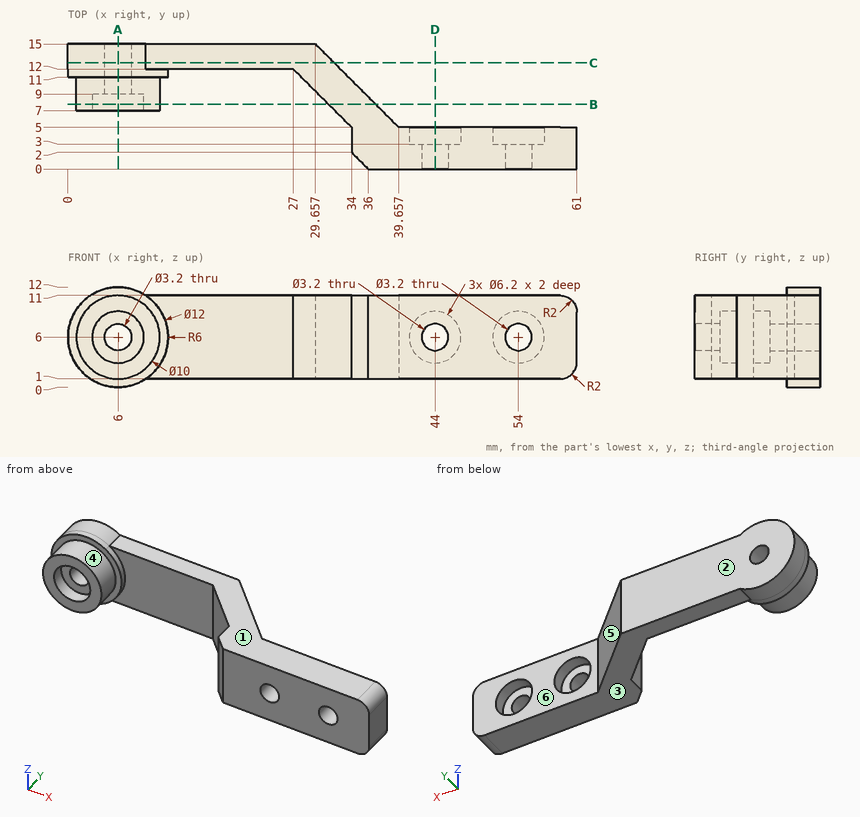
Here's the drawing with two shaded views (mm, measured from the low corner). I have some questions. A direction names the side the tool comes from. Give positions to 0.01 mm unless a question says otherwise; leave off trailing zeros. Loops run counter-clockwise (first coordinate to the right, second up) from the corner with the lowest first, then second, coordinate; pieces in that order, holes last. Notation, with made-up numbers: (52.25, -17) - (80.25, -17) arc R20 ccw to (80.25, 3) - close; hole circle Ø1 at (58.5, -7.5). An arc over 180 degrees is marked (long way). Answer in a Markdown table with one row per item. Add a question column.
Q1. For pin 1 (3 mm diameter, centred on x = 55, z = 5, fed in from +Y); pin 2 (3.5 mm diameter, centred on y = 3, z = 6, fed in from -X); pin 3 (3 mm diameter, centred on x = 4.5, z = 4, fed in from -Y), each with a flat end and sliding along its axis, tell me the tip position at first contact or that it passes through.
Q2. Please list where these lines run through material, in increasing order: L1, parallel to X at y = 3.7, z = 6; L2, parallel to Z at x = 44, y = 4.2; L3, parallel to X at y = 2.35, z = 6. Write a range as from..to.
Q3. If we section it at A-A (x = 6): List the corners of the cut face in (y, z) for me.
Q4. We'd pull the mould along X, two halves only. Please class the marked faces 4, 5 and 6: +X half, -X half, draft (parallel to the pull), parting line (faces both ways), or undercut.
Q5. If we section it at D-D (x = 44): List the corners of the cut face in (y, z) for me, plus the area to 3 significant figures.
Q6. Which directions (+Z, -Z, +X, -X, +Y, -Y) give clear straight access to the entire face, cutting with the end or side of a thin tool? Please do the marked faces 1, 2 and 3.
Q7. If we section it at B-B (y = 7.75): List the corners of the cut face in (x, z) for me.
Q8. If we section it at C-C (y = 12.75): List the corners of the cut face in (x, z) for me.
The answers:
| question | item | result |
|---|---|---|
| 1 | pin 1 | stops at y = 3 |
| 1 | pin 2 | stops at x = 34 |
| 1 | pin 3 | stops at y = 7 |
| 2 | L1 | x = 34..40.9, 47.1..50.9, 57.1..61 |
| 2 | L2 | z = 1..2.9, 9.1..11 |
| 2 | L3 | x = 34..42.4, 45.6..52.4, 55.6..61 |
| 3 | outline | (7, 1) - (11, 1) - (11, 0) - (15, 0) - (15, 4.4) - (9, 4.4) - (9, 2.9) - (7, 2.9) - close; (7, 9.1) - (9, 9.1) - (9, 7.6) - (15, 7.6) - (15, 12) - (11, 12) - (11, 11) - (7, 11) - close |
| 4 | face 4 | undercut |
| 4 | face 5 | +X half |
| 4 | face 6 | draft |
| 5 | outline | (0, 1) - (5, 1) - (5, 2.9) - (3, 2.9) - (3, 4.4) - (0, 4.4) - close; (0, 7.6) - (3, 7.6) - (3, 9.1) - (5, 9.1) - (5, 11) - (0, 11) - close |
| 5 | area | 28.0 mm^2 |
| 6 | face 1 | +Z, +X, +Y, -Y |
| 6 | face 2 | +Z, -Z, +X, -X, +Y |
| 6 | face 3 | -Z, +X, +Y, -Y |
| 7 | outline | circle Ø10 at (6, 6); (31.25, 1) - (36.91, 1) - (36.91, 11) - (31.25, 11) - close; hole circle Ø6.2 at (6, 6) |
| 8 | outline | (9.32, 1) - (31.91, 1) - (31.91, 11) - (9.32, 11) arc R6 ccw (long way) to start; hole circle Ø3.2 at (6, 6) |
